```python
from build123d import *

# Parameters (mm, degrees)
CUT_EXTRUDE3_DEPTH           = 60
CUT_EXTRUDE5_DEPTH           = 2
CUT_EXTRUDE5_DEPTH_BACK      = 30
SKETCH9_R                    = 38
SKETCH9_R_2                  = 23
SKETCH19_W                   = 12
SKETCH19_H                   = 36.5
CUT_REVOLVE2_ANGLE           = 65
CUT_REVOLVE2_OTHER_WAY_ANGLE = 65
SKETCH21_W                   = 3.25
SKETCH21_H                   = 4
BOSS_EXTRUDE3_DEPTH          = 1.35
CIRPATTERN1_COUNT            = 5
CUT_EXTRUDE9_START           = -5
CUT_EXTRUDE9_DEPTH           = 5
SKETCH23_R                   = 10.5
CUT_EXTRUDE10_DEPTH          = 10
SKETCH24_W                   = 17
SKETCH24_H                   = 12
BOSS_EXTRUDE4_DEPTH          = 8
SKETCH26_W                   = 12
SKETCH26_H                   = 8
CUT_EXTRUDE11_DEPTH          = 10
SKETCH27_W                   = 4
SKETCH27_H                   = 5
CUT_EXTRUDE12_DEPTH          = 5
CUT_EXTRUDE14_DEPTH          = 2
CUT_EXTRUDE14_DEPTH_BACK     = 30
SKETCH29_R                   = 1
CUT_EXTRUDE15_DEPTH          = 15
FILLET1_R                    = 6
FILLET2_R                    = 8
SKETCH30_W                   = 97.703590575
SKETCH30_H                   = 5
CUT_EXTRUDE16_DEPTH          = 5
INTERSECT1_DEPTH             = 20.469057744
INTERSECT1_START             = 55.427876097
INTERSECT1_2_OUTLINE_R       = 40
INTERSECT1_2_OUTLINE_W       = 12
INTERSECT1_2_OUTLINE_H       = 8
INTERSECT1_2_DEPTH           = 8
INTERSECT1_START_2           = 50.427876097
INTERSECT1_3_OUTLINE_W       = 17
INTERSECT1_3_OUTLINE_H       = 12
INTERSECT1_3_OUTLINE_W_2     = 12
INTERSECT1_3_OUTLINE_H_2     = 8
INTERSECT1_3_DEPTH           = 5


with BuildPart() as part:
    # Sketch1 → Revolve1 (revolve)
    with BuildSketch(Plane.XY, mode=Mode.PRIVATE) as revolve1_sk:
        with BuildLine():
            Line((0, 63.427876097), (32, 63.427876097))
            ThreePointArc((32, 63.427876097), (37.656854249, 61.084730346), (40, 55.427876097))
            Line((40, 55.427876097), (40, 28.846818009))
            ThreePointArc((40, 28.846818009), (38.792081772, 24.082439968), (35.460140376, 20.469057744))
            Line((35.460140376, 20.469057744), (28.539859624, 15.958818353))
            ThreePointArc((28.539859624, 15.958818353), (25.207918228, 12.345436129), (24, 7.581058088))
            Line((24, 7.581058088), (24, 3.25))
            Line((24, 3.25), (24.35, 3))
            Line((24.35, 3), (24.35, 0))
            Line((24.35, 0), (22.5, 0))
            Line((22.5, 0), (22.5, 12.5))
            ThreePointArc((22.5, 12.5), (22.353553391, 12.853553391), (22, 13))
            Line((22, 13), (0, 13))
            Line((0, 13), (0, 63.427876097))
        make_face()
    revolve(revolve1_sk.sketch.rotate(Axis((0, 0, 0), (0, 1, 0)), 90), axis=Axis((0, 0, 0), (0, 1, 0)))

    # Sketch11 → Cut-Extrude3 (cut)
    with BuildSketch(Plane(origin=(0, 13, 0), x_dir=(-1, 0, 0), z_dir=(0, -1, 0))):
        with BuildLine():
            Line((-21, 0), (21, 0))
            ThreePointArc((21, 0), (0, 21), (-21, 0))
        make_face()
    extrude(amount=-CUT_EXTRUDE3_DEPTH, mode=Mode.SUBTRACT)

    # Sketch9 → Cut-Extrude5 (cut, two sides: drawn at the far end of the back side and taken through both)
    with BuildSketch(Plane(origin=(0, 55.427876097, 0), x_dir=(1, 0, 0), z_dir=(0, 1, 0)).offset(-CUT_EXTRUDE5_DEPTH_BACK)):
        with Locations(Location((0, 0, 0), (0, 0, 270))):
            Circle(SKETCH9_R)
        with Locations(Location((0, 0, 0), (0, 0, 270))):
            Circle(SKETCH9_R_2, mode=Mode.SUBTRACT)
    extrude(amount=CUT_EXTRUDE5_DEPTH + CUT_EXTRUDE5_DEPTH_BACK, mode=Mode.SUBTRACT)

    # Sketch19 → Cut-Revolve2 (revolve, cut)
    with BuildSketch(Plane(origin=(0, 0, 0), x_dir=(0, 0, -1), z_dir=(1, 0, 0))):
        with Locations((-41.064715832, 37.177876097)):
            Rectangle(SKETCH19_W, SKETCH19_H)
    revolve(axis=Axis((0, 0, 0), (0, 1, 0)), revolution_arc=CUT_REVOLVE2_ANGLE, mode=Mode.SUBTRACT)

    # Sketch19 → Cut-Revolve2 other way (revolve, cut)
    with BuildSketch(Plane(origin=(0, 0, 0), x_dir=(0, 0, -1), z_dir=(1, 0, 0))):
        with Locations((-41.064715832, 37.177876097)):
            Rectangle(SKETCH19_W, SKETCH19_H)
    revolve(axis=Axis((0, 0, 0), (0, -1, 0)), revolution_arc=CUT_REVOLVE2_OTHER_WAY_ANGLE, mode=Mode.SUBTRACT)

    # Sketch21 → Boss-Extrude3 (add)
    with BuildSketch(Plane(origin=(0, 0, 22.5), x_dir=(-1, 0, 0), z_dir=(0, 0, -1))):
        with Locations((0, 2)):
            Rectangle(SKETCH21_W, SKETCH21_H)
    boss_extrude3 = extrude(amount=BOSS_EXTRUDE3_DEPTH)

    # CirPattern1: Boss-Extrude3 ×5 about axis
    cirpattern1_axis = Axis((0, 0, 0), (0, 1, 0))
    for i in range(1, CIRPATTERN1_COUNT):
        add(boss_extrude3.rotate(cirpattern1_axis, i * 360 / CIRPATTERN1_COUNT))

    # Cut-Extrude9: read off the stored shape, not the designer's step
    # Cut-Extrude9 outline → Cut-Extrude9 (cut)
    with BuildSketch(Plane(origin=(0, 63.427876097, 0), x_dir=(1, 0, 0), z_dir=(0, 1, 0)).offset(CUT_EXTRUDE9_START)):
        with BuildLine():
            ThreePointArc((40, 0), (0, 40), (-40, 0))
            Line((-40, 0), (-21, 0))
            ThreePointArc((-21, 0), (0, 21), (21, 0))
            Line((21, 0), (40, 0))
        make_face()
    extrude(amount=CUT_EXTRUDE9_DEPTH, mode=Mode.SUBTRACT)

    # Sketch23 → Cut-Extrude10 (cut)
    with BuildSketch(Plane(origin=(0, 0, -40), x_dir=(-1, 0, 0), z_dir=(0, 0, -1))):
        with Locations((0, 42.137876097)):
            Circle(SKETCH23_R)
    extrude(amount=-CUT_EXTRUDE10_DEPTH, mode=Mode.SUBTRACT)

    # Sketch24 → Boss-Extrude4 (add)
    with BuildSketch(Plane(origin=(0, 58.427876097, 0), x_dir=(1, 0, 0), z_dir=(0, 1, 0))):
        with Locations((0, 30)):
            Rectangle(SKETCH24_W, SKETCH24_H)
    extrude(amount=-BOSS_EXTRUDE4_DEPTH)

    # Sketch26 → Cut-Extrude11 (cut)
    with BuildSketch(Plane(origin=(0, 58.427876097, 0), x_dir=(1, 0, 0), z_dir=(0, 1, 0))):
        with Locations((0, 30)):
            Rectangle(SKETCH26_W, SKETCH26_H)
    extrude(amount=-CUT_EXTRUDE11_DEPTH, mode=Mode.SUBTRACT)

    # Sketch27 → Cut-Extrude12 (cut)
    with BuildSketch(Plane(origin=(8.5, 0, 0), x_dir=(0, 0, -1), z_dir=(1, 0, 0))):
        with Locations((29.5, 53.927876097)):
            Rectangle(SKETCH27_W, SKETCH27_H)
    extrude(amount=-CUT_EXTRUDE12_DEPTH, mode=Mode.SUBTRACT)

    # Sketch28 → Cut-Extrude14 (cut, two sides: drawn at the far end of the back side and taken through both)
    with BuildSketch(Plane(origin=(0, 55.427876097, 0), x_dir=(1, 0, 0), z_dir=(0, 1, 0)).offset(-CUT_EXTRUDE14_DEPTH_BACK)):
        with BuildLine():
            Line((-22.912878475, -2), (22.912878475, -2))
            ThreePointArc((22.912878475, -2), (0, -23), (-22.912878475, -2))
        make_face()
    extrude(amount=CUT_EXTRUDE14_DEPTH + CUT_EXTRUDE14_DEPTH_BACK, mode=Mode.SUBTRACT)

    # Sketch29 → Cut-Extrude15 (cut)
    with BuildSketch(Plane(origin=(0, 0, 0), x_dir=(-1, 0, 0), z_dir=(0, 0, -1))):
        with Locations((-30.416198487, 60.927876097)):
            Circle(SKETCH29_R)
        with Locations((30.416198487, 60.927876097)):
            Circle(SKETCH29_R)
        with Locations((0, 60.927876097)):
            Circle(SKETCH29_R)
    extrude(amount=-CUT_EXTRUDE15_DEPTH, mode=Mode.SUBTRACT)

    # Fillet1
    fillet1_edges = [part.edges().sort_by_distance(p)[0] for p in [
        (21, 35.713938048, 0),
        (-21, 35.713938048, 0),
    ]]
    fillet(fillet1_edges, radius=FILLET1_R)

    # Fillet2
    fillet2_edges = [part.edges().sort_by_distance(p)[0] for p in [
        (-22.912878475, 41.427876097, 2),
        (22.912878475, 41.427876097, 2),
    ]]
    fillet(fillet2_edges, radius=FILLET2_R)

    # Sketch30 → Cut-Extrude16 (cut)
    with BuildSketch(Plane(origin=(0, 63.427876097, 0), x_dir=(1, 0, 0), z_dir=(0, 1, 0))):
        with Locations((-0.528699084, -2.5)):
            Rectangle(SKETCH30_W, SKETCH30_H)
    extrude(amount=-CUT_EXTRUDE16_DEPTH, mode=Mode.SUBTRACT)

    # Intersect1: read off the stored shape, not the designer's step
    # Intersect1 outline → Intersect1 (cut)
    with BuildSketch(Plane(origin=(0, 0, 0), x_dir=(1, 0, 0), z_dir=(0, 1, 0))):
        with BuildLine():
            Line((31.779425009, -14.818989253), (32.137801352, -14.986102887))
            ThreePointArc((32.137801352, -14.986102887), (0, 35.460140376), (-32.137801352, -14.986102887))
            Line((-32.137801352, -14.986102887), (-31.779425009, -14.818989253))
            ThreePointArc((-31.779425009, -14.818989253), (0, -35.064715832), (31.779425009, -14.818989253))
        make_face()
        with BuildLine():
            ThreePointArc((-13.747727085, 0), (-18.767687244, 2.713664655), (-19.246817919, 8.4))
            ThreePointArc((-19.246817919, 8.4), (0, 21), (19.246817919, 8.4))
            ThreePointArc((19.246817919, 8.4), (18.767687244, 2.713664655), (13.747727085, 0))
            Line((13.747727085, 0), (-13.747727085, 0))
        make_face(mode=Mode.SUBTRACT)
    extrude(amount=INTERSECT1_DEPTH, mode=Mode.SUBTRACT)

    # Intersect1 2 outline → Intersect1 2 (cut)
    with BuildSketch(Plane(origin=(0, 0, 0), x_dir=(1, 0, 0), z_dir=(0, 1, 0)).offset(INTERSECT1_START)):
        Circle(INTERSECT1_2_OUTLINE_R)
        with Locations((0, 30)):
            Rectangle(INTERSECT1_2_OUTLINE_W, INTERSECT1_2_OUTLINE_H, mode=Mode.SUBTRACT)
        with BuildLine():
            ThreePointArc((-13.747727085, 0), (-18.767687244, 2.713664655), (-19.246817919, 8.4))
            ThreePointArc((-19.246817919, 8.4), (0, 21), (19.246817919, 8.4))
            ThreePointArc((19.246817919, 8.4), (18.767687244, 2.713664655), (13.747727085, 0))
            Line((13.747727085, 0), (-13.747727085, 0))
        make_face(mode=Mode.SUBTRACT)
    extrude(amount=INTERSECT1_2_DEPTH, mode=Mode.SUBTRACT)

    # Intersect1 3 outline → Intersect1 3 (cut)
    with BuildSketch(Plane(origin=(0, 0, 0), x_dir=(1, 0, 0), z_dir=(0, 1, 0)).offset(INTERSECT1_START_2)):
        with Locations((0, 30)):
            Rectangle(INTERSECT1_3_OUTLINE_W, INTERSECT1_3_OUTLINE_H)
        with Locations((0, 30)):
            Rectangle(INTERSECT1_3_OUTLINE_W_2, INTERSECT1_3_OUTLINE_H_2, mode=Mode.SUBTRACT)
    extrude(amount=INTERSECT1_3_DEPTH, mode=Mode.SUBTRACT)


solid = part.part
```
The model under review builds one solid part; all positions refer to its coordinate system, in mm. A direction names the side the tool comes from. Round coordinates to 2 decimals unless told otherwise and drop trailing zeros. Loops run counter-clockwise (first coordinate to the right, second up) from the corner with the lowest first, then second, coordinate; pieces in that order, holes last. Notation, with made-up numbers: (18, 12) - (71, 12) arc R17 cw to (71, 33) - close; hole circle Ø11 at (78.5, 62.25). An arc over 180 degrees is marked (long way). Use a Markdown table: item, result. Add a question column.
Q1. Add section B-B (x = 0). State the section outline as (y, z) points.
Q2. Add section A-A (y = 46). State the section outline as (x, z) points.
Q3. Machinability: for faces 4 (the face through (0, 40, -23)), 5 (the face through (18.72, 38.19, -2.64)), 6 (the face through (0, 40, 2)), which of the approach directions +Z, -Z, +X, -X, +Y, -Y give a long, thin tool a straight path to every point of the face, cutting with its end or side? Answer none if there is none.
Q4. Add section D-D (z = 23). State the section outline as (x, y) points.
Q5. Insertion check: pin 1 Ø12 at (x, z) = (-28.5, -12) entering from +Y; pin 2 Ø10 at (y, z) = (33.5, -9.5) entering from -X; pin 3 Ø8 at (x, y) = (-6.5, 39.5) entering from +Z. Each pin has a flat end and moves straight along its axis. Give the tip position at first contact, or say it passes through.
Q6. Add section C-C (y = 37.5). State the section outline as (x, z) points, plus the area to 3 significant figures.
Q7. For probe 1 along Z at (x, y) = (-13, 28.5); probe 2 along X at (y, z) = (27, -17); probe 3 along Z at (x, y) = (1, 29), list the stretches that pass through material, from the lowest coordinate up.
Q8. The part is to be moulded in two halves that separate along X. For faces 1 (the face through (-16.23, 41.95, -36.56)), 2 (the face through (0, 38, 0)), 3 (the face through (0, 55.428, 1)), say which applies: pulls with the +X half, pulls with the -X half, needs draft (parallel to the pull), parting line crosses it, or undercut.
Worked answers:
| question | item | result |
|---|---|---|
| 1 | outline | (20.47, -35.46) arc R10 ccw to (28.85, -40) - (31.64, -40) - (31.64, -38) - (25.43, -38) - (25.43, -23) - (55.43, -23) - (55.43, -21) - (20.47, -21) - close; (20.47, 0) - (55.43, 0) - (55.43, 2) - (25.43, 2) - (25.43, 35.06) - (20.47, 35.06) - close; (52.64, -40) - (55.43, -40) - (55.43, -38) - (52.64, -38) - close |
| 2 | outline | (-36.25, 16.9) arc R40 ccw to (-9.76, -38.79) - (-9.76, -36.72) arc R38 cw to (-34.44, 16.06) - close; (-21.08, -9.2) arc R23 ccw to (21.08, -9.2) arc R8 ccw to (13.75, 2) - (-13.75, 2) arc R8 ccw to start; (9.76, -38.79) arc R40 ccw to (36.25, 16.9) - (34.44, 16.06) arc R38 cw to (9.76, -36.72) - close; hole (-19.25, -8.4) arc R21 ccw to (19.25, -8.4) arc R6 ccw to (13.75, 0) - (-13.75, 0) arc R6 ccw to start |
| 3 | face 4 | +Y |
| 3 | face 5 | +Y, -Y |
| 3 | face 6 | +Z, +Y |
| 4 | outline | (-26.47, 20.47) - (26.47, 20.47) - (26.47, 25.43) - (-26.47, 25.43) - close |
| 5 | pin 1 | y = 25.43 |
| 5 | pin 2 | x = -39.75 |
| 5 | pin 3 | z = 2 |
| 6 | outline | (-36.25, 16.9) arc R40 ccw to (-9.42, -38.87) - (-9.42, -36.81) arc R38 cw to (-34.44, 16.06) - close; (-21.08, -9.2) arc R23 ccw to (21.08, -9.2) arc R8 ccw to (13.75, 2) - (-13.75, 2) arc R8 ccw to start; (9.42, -38.87) arc R40 ccw to (36.25, 16.9) - (34.44, 16.06) arc R38 cw to (9.42, -36.81) - close; hole (-19.25, -8.4) arc R21 ccw to (19.25, -8.4) arc R6 ccw to (13.75, 0) - (-13.75, 0) arc R6 ccw to start |
| 6 | area | 488 mm² |
| 7 | probe 1 | -37.82 to -35.71, -18.97 to -16.49, 0 to 2 |
| 7 | probe 2 | -36.02 to -33.99, -15.49 to -12.33, 12.33 to 15.49, 33.99 to 36.02 |
| 7 | probe 3 | -39.99 to -37.99, -22.98 to -20.98, 0 to 2 |
| 8 | face 1 | parting line crosses it |
| 8 | face 2 | undercut |
| 8 | face 3 | needs draft |
